Solid Edge part; units mm, degrees
sketch "Sketch1" plane through (0, 0, 0) normal (0, 0, 1) x (1, 0, 0)
  line L0 (-13.35, -3.75) -> (13.35, -3.75)
  line L1 (13.35, -3.75) -> (13.35, 3.75)
  line L2 (13.35, 3.75) -> (-13.35, 3.75)
  line L3 (-13.35, 3.75) -> (-13.35, -3.75)
  dimension "D1" = 13.35
  dimension "D2" = 13.35
extrude "Protrusion1" add sketch "Sketch1" along normal mid plane 4.7
fillet "Verrundung_1" radius 3.75 4 edges at (13.35, -3.75, 0) (13.35, 3.75, 0) (-13.35, -3.75, 0) (-13.35, 3.75, 0)
sketch "Sketch2" plane through (0, 0, 2.35) normal (0, 0, 1) x (1, 0, 0)
  line L0 (-9.6, -2.75) -> (9.6, -2.75)
  arc A0 (9.6, -2.75) -> (12.35, 0) centre (9.6, 0) ccw
  arc A1 (12.35, 0) -> (9.6, 2.75) centre (9.6, 0) ccw
  line L1 (9.6, 2.75) -> (-9.6, 2.75)
  arc A2 (-9.6, 2.75) -> (-12.35, 0) centre (-9.6, 0) ccw
  arc A3 (-9.6, -2.75) -> (-12.35, 0) centre (-9.6, 0) cw
  dimension "D1" = 9.6
extrude "Extrusionsausschnitt_1" cut sketch "Sketch2" against normal blind 1.2 flip side to cut
sketch "Sketch3" plane through (0, 0, -2.35) normal (0, 0, -1) x (1, 0, 0)
  line L0 (-9.6, -2.75) -> (9.6, -2.75)
  arc A0 (9.6, -2.75) -> (12.35, 0) centre (9.6, 0) ccw
  arc A1 (12.35, 0) -> (9.6, 2.75) centre (9.6, 0) ccw
  line L1 (9.6, 2.75) -> (-9.6, 2.75)
  arc A2 (-9.6, 2.75) -> (-12.35, 0) centre (-9.6, 0) ccw
  arc A3 (-9.6, -2.75) -> (-12.35, 0) centre (-9.6, 0) cw
  dimension "D1" = 9.6
extrude "Extrusionsausschnitt_2" cut sketch "Sketch3" against normal blind 2.5 flip side to cut
sketch "Sketch4" plane through (0, 0, 2.35) normal (0, 0, 1) x (1, 0, 0)
  line L0 (-4.76, -1.76) -> (6.52, -1.76)
  line L1 (6.52, -1.76) -> (6.52, 1.76)
  line L2 (6.52, 1.76) -> (-4.76, 1.76)
  arc A0 (-4.76, 1.76) -> (-6.52, 0) centre (-4.76, 0) ccw
  arc A1 (-4.76, -1.76) -> (-6.52, 0) centre (-4.76, 0) cw
  dimension "D1" = 6.52
  dimension "D2" = 6.52
extrude "Extrusionsausschnitt_3" cut sketch "Sketch4" against normal blind 1.2
sketch "Sketch5" plane through (0, 0, 1.15) normal (0, 0, 1) x (1, 0, 0)
  circle A0 centre (4.4, 0) radius 0.3
  circle A1 centre (2.2, 0) radius 0.3
  circle A2 centre (0, 0) radius 0.3
  circle A3 centre (-2.2, 0) radius 0.3
  circle A4 centre (-4.4, 0) radius 0.3
extrude "Extrusionsausprägung_2" add sketch "Sketch5" along normal blind 1.2 and the other way blind 5
fillet "Verrundung_2" radius 0.1 11 edges at (0.88, 1.76, 2.35) (-6.52, 0, 2.35) (0.88, -1.76, 2.35) (6.52, 0, 2.35) (0, 2.75, 2.35) (-12.35, 0, 2.35) (0, -2.75, 2.35) (12.35, 0, 2.35) (0, 3.75, 1.15) (-13.35, 0, 1.15) (0, -3.75, 1.15)
Verification items for the finished model (mm, model axes). A direction names the side the tool comes from. Give positions to 0.01 mm unless a question says otherwise; leave off trailing zeros. Loops run counter-clockwise (first coordinate to the right, second up) from the corner with the lowest first, then second, coordinate; pieces in that order, holes last.
1) Set-up check for faces 5 (the flat face through (0, -2.75, -1)), 6 (the cylindrical face through (12.35, 0.06, -1.12)), 7 (the flat face through (0, 3, 1.15)), 8 (the cylindrical face through (-12.35, 0.06, 1.71)), 9 (the flat face through (0, -2.75, 2)): record each of +Z, -Z, +X, -X, +Y, -Y from which the full face is reachable in a straight line by a thin tool's end or side.
2) Sectioned sample at C-C, the plane z = -2.75. Enter the section's corners in (x, y).
3) Draft check along X on faces 1 (the flat face through (0, 2.75, 2)), 2 (the flat face through (1, 1.76, 2)), 3 (the cylindrical face through (12.2, -2.7, 0.6)), 4 (the cylindrical face through (-12.35, -0.06, -1.12)). Enter one of: pulls with the +X half, pulls with the -X half, needs draft (parallel to the pull), parting line crosses it, or undercut.
4) Sectioned sample at A-A, the plane z = 1.5. Enter the section's corners in (x, y), then the cut area to 3 significant figures.
5) Sectioned sample at B-B, the plane x = -8.75. Enter the section's corners in (y, z), then the cut area to 3 significant figures.
6) Depth check by flat-ended pin: pin 1 Ø3 at (x, z) = (-2.5, -1.5) entering from -Y; pin 2 Ø1 at (x, y) = (-3.5, 0.5) entering from -Z; pin 3 Ø1.5 at (x, z) = (-4.5, -1) entering from +Y. Enter the tip coordinate at first touch or a pass-through.
7) Sectioned sample at D-D, the plane x = 5.25. Enter the section's corners in (y, z), then the cut area to 3 significant figures.
8) Thickness scan on line 1 along Y through (x, z) = (2.25, 1.5); line 2 along Z through (x, y) = (-7.5, 0.75); line 3 along Z through (x, y) = (-6, 3.25). Record the ranges inside material, lowest first.
Answers:
1. face 5: -Z, +X, -X, -Y
1. face 6: -Z, +X
1. face 7: +Z
1. face 8: +Z, -X
1. face 9: +Z, +X, -X, -Y
2. outline: circle Ø0.6 at (-4.4, 0); circle Ø0.6 at (-2.2, 0); circle Ø0.6 at (0, 0); circle Ø0.6 at (2.2, 0); circle Ø0.6 at (4.4, 0)
3. face 1: needs draft
3. face 2: undercut
3. face 3: pulls with the +X half
3. face 4: pulls with the -X half
4. outline: (-9.6, -2.75) - (9.6, -2.75) arc R2.75 ccw to (9.6, 2.75) - (-9.6, 2.75) arc R2.75 ccw to start; circle Ø0.6 at (-4.4, 0); circle Ø0.6 at (-2.2, 0); circle Ø0.6 at (0, 0); circle Ø0.6 at (2.2, 0); circle Ø0.6 at (4.4, 0); hole (-4.76, -1.76) - (6.52, -1.76) - (6.52, 1.76) - (-4.76, 1.76) arc R1.76 ccw to start
4. area: 86.2 mm2
5. outline: (-3.75, 0.15) - (-2.75, 0.15) - (-2.75, -2.35) - (2.75, -2.35) - (2.75, 0.15) - (3.75, 0.15) - (3.75, 1.05) arc R0.1 ccw to (3.65, 1.15) - (2.75, 1.15) - (2.75, 2.25) arc R0.1 ccw to (2.65, 2.35) - (-2.65, 2.35) arc R0.1 ccw to (-2.75, 2.25) - (-2.75, 1.15) - (-3.65, 1.15) arc R0.1 ccw to (-3.75, 1.05) - close
5. area: 27.8 mm2
6. pin 1: stops at y = -2.75
6. pin 2: stops at z = -2.35
6. pin 3: stops at y = 2.75
7. outline: (-3.75, 0.15) - (-2.75, 0.15) - (-2.75, -2.35) - (2.75, -2.35) - (2.75, 0.15) - (3.75, 0.15) - (3.75, 1.05) arc R0.1 ccw to (3.65, 1.15) - (2.75, 1.15) - (2.75, 2.25) arc R0.1 ccw to (2.65, 2.35) - (1.86, 2.35) arc R0.1 ccw to (1.76, 2.25) - (1.76, 1.15) - (-1.76, 1.15) - (-1.76, 2.25) arc R0.1 ccw to (-1.86, 2.35) - (-2.65, 2.35) arc R0.1 ccw to (-2.75, 2.25) - (-2.75, 1.15) - (-3.65, 1.15) arc R0.1 ccw to (-3.75, 1.05) - close
7. area: 23.6 mm2
8. line 1: y = -2.75 to -1.76, -0.3 to 0.3, 1.76 to 2.75
8. line 2: z = -2.35 to 2.35
8. line 3: z = 0.15 to 1.15
